The listing builds one solid part. Answer for the finished solid, in the listing's coordinates (mm). A direction names the side the tool comes from. Coordinates: 2 decimals unless noted, no trailing zeros. Loops run counter-clockwise (first coordinate to the right, second up) from the corner with the lowest first, then second, coordinate; pieces in that order, holes last. Notation, with made-up numbers: M 54,23 L 111,23 A14 cw 111,27 Z; hole C 69,-31.5 d2. An arc over 180 degrees is marked long. Return JSON: item names as keys, results as strings. Group by question number.
1. The mould has two halves that part along X. Classify faces 6 (the face through (62, -2, 50)), 7 (the face through (2, -2, 25)), 8 (the face through (135, -2, -2)): pulls with the +X half, pulls with the -X half, needs draft (parallel to the pull), parting line crosses it, or undercut.
2. Section C-C (x = 59.5) is taken. Write down the section's boundary in (y, z).
3. Straight lines are drawn through the part: L1, parallel to Z at x = 11, y = -2.25; L2, parallel to X at y = -0.35, z = 26.5. For each, find the intervals that lie inside material, in ascending order. Write a range as from..to.
4. Which of the six approach directions +Z, -Z, +X, -X, +Y, -Y give full straight-line access (tool end or side, diameter ignored) to faces 1 (the face through (13, -2, 0)), 2 (the face through (62, -2, 0)), 3 (the face through (142, -2, 25)), 4 (the face through (112, -2, 50)), 5 (the face through (14, -2, 50))?
5. Section B-B (z = 24.5) is taken. Write down the section's boundary in (x, y).
6. Given P1, Ø1.6, axis at x = 1, y = -2, coming from the -Z side; P2, Ø2, axis at x = 73, y = -4.5, coming from the +Z side; P3, Ø1.6, axis at y = -3.5, z = -1, coming from the -X side, each flat-ended and moving along its own axis, determine where each tip first touches the part or whether it passes through.
```python
from build123d import *

# Parameters (mm, degrees)
F1_DEPTH = 5


with BuildPart() as f1:
    # F0 (on Front) → F1 (new body)
    with BuildSketch(Plane.XZ):
        Polygon((0, 15), (0, 0), (27, 0), (27, -2), (47, -2), (47, 0), (77, 0), (77, -2), (97, -2), (97, 0), (127, 0), (127, -2), (144, -2), (144, 15), (142, 15), (142, 35), (144, 35), (144, 52), (127, 52), (127, 50), (97, 50), (97, 52), (77, 52), (77, 50), (47, 50), (47, 52), (27, 52), (27, 50), (0, 50), (0, 35), (2, 35), (2, 15), align=None)
    extrude(amount=F1_DEPTH)


solid = f1.part
```
Worked out:
{
 "1": {"face 6": "undercut", "face 7": "pulls with the -X half", "face 8": "needs draft"},
 "2": {"outline": "M -5,0 L 0,0 L 0,50 L -5,50 Z"},
 "3": {"L1": "0..50", "L2": "2..142"},
 "4": {"face 1": "-Z, -X, +Y, -Y", "face 2": "-Z, +Y, -Y", "face 3": "+X, +Y, -Y", "face 4": "+Z, +Y, -Y", "face 5": "+Z, -X, +Y, -Y"},
 "5": {"outline": "M 2,-5 L 142,-5 L 142,0 L 2,0 Z"},
 "6": {"P1": "z = 0", "P2": "z = 50", "P3": "x = 27"}
}
